Check sheet for the modelled part. Datum: model origin and axes. Units: mm. A direction names the side the tool comes from. Coordinates: 2 decimals unless noted, no trailing zeros. Loops run counter-clockwise (first coordinate to the right, second up) from the corner with the lowest first, then second, coordinate; pieces in that order, holes last. Notation, with made-up numbers: M 20.5,60 L 52.5,60 A26 cw 52.5,94 Z; hole C 45,26.25 d11. An arc over 180 degrees is marked long. Return JSON: item names as keys, results as strings.
Autodesk Inventor part; units mm, degrees
ref_plane "Start Plane" through (0, 0, 0) normal (0, 0, 1) x (1, 0, 0)
ref_plane "End Plane" through (0, 0, 119.1864) normal (0, 0, 1) x (1, 0, 0)
ref_plane "Work Plane6" through (223.7362, -9.1535, 95.5954) normal (0, -0.851, 0.5252) x (1, 0, 0)
ref_plane "Start Plane" through (0, 0, 0) normal (0, 0, 1) x (1, 0, 0)
ref_plane "End Plane" through (0, 0, 119.1864) normal (0, 0, 1) x (1, 0, 0)
sketch "Sketch" plane through (0, 0, 0) normal (0, 0, 1) x (1, 0, 0)
  line L0 (-10, -7) -> (-10, 7)
  line L1 (-7, 10) -> (7, 10)
  line L2 (10, 7) -> (10, -7)
  line L3 (7, -10) -> (-7, -10)
  arc A0 (-10, -7) -> (-7, -10) centre (-7, -7) ccw
  arc A1 (-7, 10) -> (-10, 7) centre (-7, 7) ccw
  arc A2 (10, 7) -> (7, 10) centre (7, 7) ccw
  arc A3 (7, -10) -> (10, -7) centre (7, -7) ccw
  arc A4 (-7, 8) -> (-8, 7) centre (-7, 7) ccw
  line L4 (-7, 8) -> (7, 8)
  arc A5 (8, 7) -> (7, 8) centre (7, 7) ccw
  line L5 (8, 7) -> (8, -7)
  arc A6 (7, -8) -> (8, -7) centre (7, -7) ccw
  line L6 (7, -8) -> (-7, -8)
  arc A7 (-8, -7) -> (-7, -8) centre (-7, -7) ccw
  line L7 (-8, -7) -> (-8, 7)
  line L8 (0, 14.8698) -> (0, -14.8698) construction
  line L9 (-14.8698, 0) -> (14.8698, 0) construction
  dimension "d7" = 3
  dimension "d10" = 20
  dimension "d11" = 20
  dimension "d12" = 2
  dimension "d15" = 10
  dimension "d16" = 10
extrude "Body" add sketch "Sketch" along normal up to surface (119.1864 mm away) from surface at 0
sketch "Sketch3" plane through (0, 0, 0) normal (0, 0, 1) x (1, 0, 0)
  line L0 (0, 0) -> (10, 0)
ref_plane "Work Plane3" through (0, 0, 0) normal (0, -1, 0) x (1, 0, 0)
sketch "Sketch4" plane through (0, 0, 0) normal (0, -1, 0) x (1, 0, 0)
  line L0 (-2, 0) -> (12, 0)
  line L1 (-2, 119.1864) -> (12, 119.1864)
  dimension "d18" = 119.1864
ref_plane "Work Plane5" through (-3.5, 10, 0) normal (0, -0.5252, -0.851) x (1, 0, 0)
ref_plane "Work Plane4" through (-4.3884, -35.4353, -90.7271) normal (0, -0.851, 0.5252) x (-0.999, 0.024, 0.0389)
split "Split1" plane through (-3.5, 10, 0) removes the side toward (0, -0.5252, -0.851)
ref_plane "Work Plane6" through (223.7362, -9.1535, 95.5954) normal (0, -0.851, 0.5252) x (1, 0, 0)
split "Split2" plane through (223.7362, -9.1535, 95.5954) removes the side toward (0, -0.851, 0.5252)
ref_plane "Work Plane7" through (224.514, -2.7866, 111.6222) normal (0.0458, 0.5247, 0.8501) x (0.9989, -0.013, -0.0458)
split "Split3" plane through (224.514, -2.7866, 111.6222) removes the side toward (0.0458, 0.5247, 0.8501)
equation "\"d7\" = G_IR"
equation "\"d10\" = G_H"
equation "\"d11\" = G_W"
equation "\"d12\" = G_T"
equation "\"d15\" = 0.5 * d10"
equation "\"d16\" = 0.5 * d11"
equation "\"d3\" = G_L"
equation "\"G_W\" = 20"
equation "\"G_H\" = 20"
equation "\"G_T\" = 2"
equation "\"G_IR\" = 3"
equation "\"G_L\" = d18"
equation "\"G_OFFSET_START\" = 0"
equation "\"G_OFFSET_END\" = 8.90098"
equation "\"d14\" = G_OFFSET_END + B_L"
equation "\"B_L\" = 110.28541"
properties part number "ISO 12633-2 - 20x20x2 - 119.19" material "Steel, Mild"
1) Go/stop test with a flat-tipped pin: pin 1 Ø6 at (x, y) = (-8, -7.5) entering from +Z. Record where the tip stops, or that it passes through.
Answers:
{"pin 1": "z = 103.14"}
2) Draft check along X on faces 1 (the face through (9.1, 9.14, 57.75)), 2 (the face through (8, 0, 59)), 3 (the face through (8.749, 0.14, 6.085)). Enter one of: +X half, -X half, draft (parallel to the pull), parting line (faces both ways), or undercut.
Answers:
{"face 1": "+X half", "face 2": "undercut", "face 3": "draft"}
3) Section check A-A on y = -5.5. Record the cut outline in (x, z), then the cut area to 3 significant figures.
Answers:
{"outline": "M -10,9.57 L -8,9.57 L -8,101.52 L -10,101.52 Z; M 8,9.57 L 10,9.57 L 10,101.52 L 8,101.52 Z", "area": "368 mm²"}
4) Section check B-B on x = -3.5. Record the cut outline in (y, z).
Answers:
{"outline": "M -10,12.34 L -8,11.11 L -8,97.46 L -10,94.22 Z; M 8,1.23 L 10,0 L 10,116.01 L 8,117.25 Z"}
5) Scan lines: line 1 along X through (y, z) = (3.75, 95); line 2 along Y through (x, z) = (7.5, 27.5). Record each from-to range of solid material in increasing order. Write a range as [from, to].
Answers:
{"line 1": "[-10, -8], [8, 10]", "line 2": "[-9.96, -7.87], [7.87, 9.96]"}
6) Section check C-C on z = 23.5. Record the cut outline in (x, y).
Answers:
{"outline": "M -10,-7 A3 ccw -7,-10 L 7,-10 A3 ccw 10,-7 L 10,7 A3 ccw 7,10 L -7,10 A3 ccw -10,7 Z; hole M -8,-7 A1 ccw -7,-8 L 7,-8 A1 ccw 8,-7 L 8,7 A1 ccw 7,8 L -7,8 A1 ccw -8,7 Z"}
7) Set-up check for faces 4 (the face through (-0.14, 8.19, 116.95)), 5 (the face through (0, 8, 59)): record each of +Z, -Z, +X, -X, +Y, -Y from which the full face is reachable in a straight line by a thin tool's end or side.
Answers:
{"face 4": "+Z, +X, +Y", "face 5": "+Z, -Z"}
